Check sheet for the modelled part. Datum: model origin and axes. Units: mm. A direction names the side the tool comes from. Coordinates: 2 decimals unless noted, no trailing zeros. Loops run counter-clockwise (first coordinate to the right, second up) from the corner with the lowest first, then second, coordinate; pieces in that order, holes last. Notation, with made-up numbers: M 42.25,7.25 L 55.25,7.25 A26 cw 55.25,38.25 Z; hole C 56,81 d5. An arc over 180 degrees is marked long. Return JSON: item names as keys, results as strings.
from build123d import *

# Parameters (mm, degrees)
SKETCH1_W                = 71.12
SKETCH1_H                = 101.6
BOSS_EXTRUDE1_DEPTH      = 6.35
SKETCH2_R                = 3.175
CUT_EXTRUDE2_DEPTH       = 6.35
BOSS_EXTRUDE2_DEPTH      = 40
SKETCH4_R                = 2.921
BOSS_EXTRUDE4_DEPTH      = 38.1
FILLET1_R                = 2.54
BOSS_EXTRUDE5_DEPTH      = 38.1
BOSS_EXTRUDE5_DEPTH_BACK = 46.35
SKETCH5_W                = 71.12
SKETCH5_H                = 6.35
SKETCH8_W                = 71.12
SKETCH8_H                = 3.175
BOSS_EXTRUDE6_DEPTH      = 6.35


with BuildPart() as part:
    # Sketch1 → Boss-Extrude1 (new body)
    with BuildSketch(Plane.XY):
        Rectangle(SKETCH1_W, SKETCH1_H)
    extrude(amount=BOSS_EXTRUDE1_DEPTH)

    # Sketch2 → Cut-Extrude2 (cut)
    with BuildSketch(Plane.XY.offset(6.35)):
        with Locations((22.86, -1.27)):
            Circle(SKETCH2_R)
    extrude(amount=-CUT_EXTRUDE2_DEPTH, mode=Mode.SUBTRACT)

    # Sketch6 → Boss-Extrude2 (add)
    with BuildSketch(Plane(origin=(0, 0, 0), x_dir=(-1, 0, 0), z_dir=(0, 0, -1))):
        Polygon((-35.56, 50.8), (-35.56, 21.23), (-0.36, 21.23), (-0.36, -23.77), (-35.56, -23.77), (-35.56, -50.8), (35.56, -50.8), (35.56, 50.8), align=None)
    extrude(amount=BOSS_EXTRUDE2_DEPTH)

    # Sketch4 → Boss-Extrude4 (add)
    with BuildSketch(Plane.XY.offset(6.35)):
        with Locations(Location((-22.86, -1.27, 0), (0, 0, 180))):
            Circle(SKETCH4_R)
    extrude(amount=BOSS_EXTRUDE4_DEPTH)

    # Fillet1
    fillet1_edges = [part.edges().sort_by_distance(p)[0] for p in [
        (-19.939, -1.27, 6.35),
    ]]
    fillet(fillet1_edges, radius=FILLET1_R)

    # Sketch5 → Boss-Extrude5 (add, two sides: drawn at the far end of the back side and taken through both)
    with BuildSketch(Plane.XY.offset(6.35).offset(-BOSS_EXTRUDE5_DEPTH_BACK)):
        with Locations((0, -53.975)):
            Rectangle(SKETCH5_W, SKETCH5_H)
    extrude(amount=BOSS_EXTRUDE5_DEPTH + BOSS_EXTRUDE5_DEPTH_BACK)

    # Sketch8 → Boss-Extrude6 (add)
    with BuildSketch(Plane(origin=(0, -50.8, 0), x_dir=(1, 0, 0), z_dir=(0, 1, 0))):
        with Locations((0, -23.8125)):
            Rectangle(SKETCH8_W, SKETCH8_H)
        with Locations((0, -40.9575)):
            Rectangle(SKETCH8_W, SKETCH8_H)
    extrude(amount=BOSS_EXTRUDE6_DEPTH)


solid = part.part
1) Draft check along Y on faces 4 (the face through (0, -54, 44.45)), 5 (the face through (18, 21.23, -20)), 6 (the face through (0, 50.8, -17)). Enter one of: +Y half, -Y half, draft (parallel to the pull), parting line (faces both ways), or undercut.
Answers:
{"face 4": "draft", "face 5": "undercut", "face 6": "+Y half"}
2) Set-up check for faces 1 (the face through (-23, -1, 44.45)), 2 (the face through (18, -23.77, -20)), 3 (the face through (-25.646, -2.147, 26.421)): record each of +Z, -Z, +X, -X, +Y, -Y from which the full face is reachable in a straight line by a thin tool's end or side.
Answers:
{"face 1": "+Z, +X, -X, +Y, -Y", "face 2": "-Z, +X", "face 3": "+Z"}
3) Scan lines: line 1 along X through (y, z) = (-1, 2); line 2 along Y through (x, z) = (22.86, 3.25) (3 decimals); line 3 along Y through (x, z) = (28.5, -21). Record each from-to range of solid material in increasing order. Write a range as [from, to].
Answers:
{"line 1": "[-35.56, 19.7], [26.02, 35.56]", "line 2": "[-57.15, -4.445], [1.905, 50.8]", "line 3": "[-57.15, -23.77], [21.23, 50.8]"}
4) Go/stop test with flat-tipped pins: pin 1 Ø8 at (x, y) = (25, 0.5) entering from +Z; pin 2 Ø8 at (x, z) = (8, 11.5) entering from +Y; pin 3 Ø1 at (x, y) = (11, 7) entering from -Z. Record where each tip stops, or that it passes through.
Answers:
{"pin 1": "z = 6.35", "pin 2": "y = -50.8", "pin 3": "z = 0"}
5) Section check D-D on x = -22.86. Record the cut outline in (y, z) (3 decimals), then the cut area to 3 significant figures.
Answers:
{"outline": "M -57.15,-40 L 50.8,-40 L 50.8,6.35 L 4.191,6.35 A2.54 cw 1.651,8.89 L 1.651,44.45 L -4.191,44.45 L -4.191,8.89 A2.54 cw -6.731,6.35 L -50.8,6.35 L -50.8,22.225 L -44.45,22.225 L -44.45,25.4 L -50.8,25.4 L -50.8,39.37 L -44.45,39.37 L -44.45,42.545 L -50.8,42.545 L -50.8,44.45 L -57.15,44.45 Z", "area": "5,510 mm²"}
6) Section check C-C on z = -26. Record the cut outline in (x, y), then the cut area to 3 significant figures.
Answers:
{"outline": "M -35.56,-57.15 L 35.56,-57.15 L 35.56,-23.77 L 0.36,-23.77 L 0.36,21.23 L 35.56,21.23 L 35.56,50.8 L -35.56,50.8 Z", "area": "6,090 mm²"}
7) Section check A-A on y = -1.27. Record the cut outline in (x, z) (3 decimals).
Answers:
{"outline": "M -35.56,-40 L 0.36,-40 L 0.36,0 L 19.685,0 L 19.685,6.35 L -17.399,6.35 A2.54 cw -19.939,8.89 L -19.939,44.45 L -25.781,44.45 L -25.781,8.89 A2.54 cw -28.321,6.35 L -35.56,6.35 Z; M 26.035,0 L 35.56,0 L 35.56,6.35 L 26.035,6.35 Z"}
8) Section check B-B on x = 22.86. Record the cut outline in (y, z) (3 decimals).
Answers:
{"outline": "M -57.15,-40 L -23.77,-40 L -23.77,0 L -4.445,0 L -4.445,6.35 L -50.8,6.35 L -50.8,22.225 L -44.45,22.225 L -44.45,25.4 L -50.8,25.4 L -50.8,39.37 L -44.45,39.37 L -44.45,42.545 L -50.8,42.545 L -50.8,44.45 L -57.15,44.45 Z; M 1.905,0 L 21.23,0 L 21.23,-40 L 50.8,-40 L 50.8,6.35 L 1.905,6.35 Z"}
